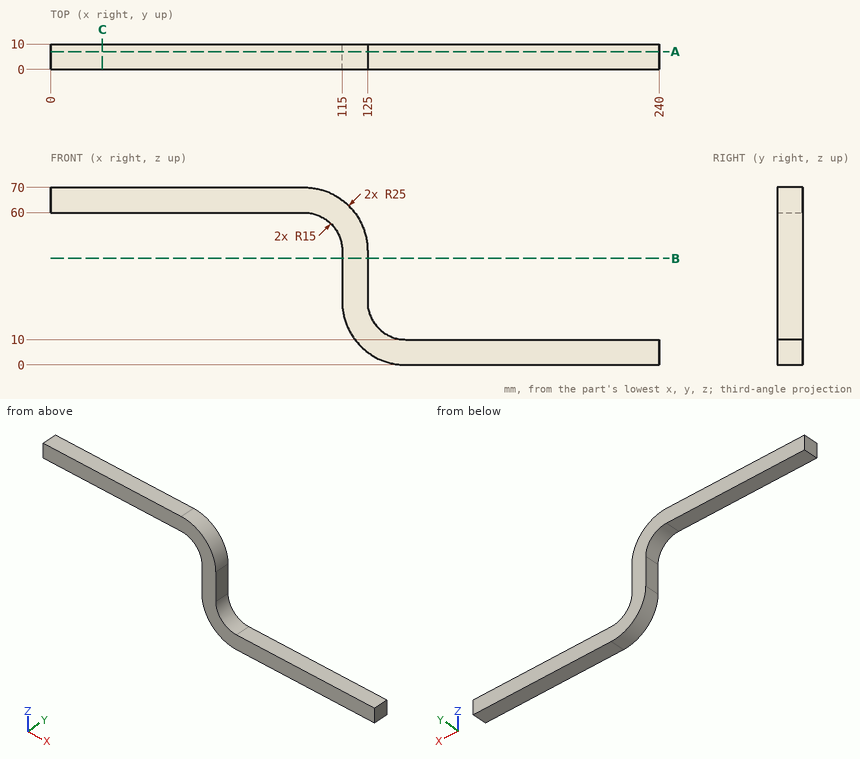
Source: three-view drawing plus pictorial views. Frame: mm from the lowest corner of the part. Round coordinates to 2 decimals unless told otherwise and drop trailing zeros. Loops run counter-clockwise (first coordinate to the right, second up) from the corner with the lowest first, then second, coordinate; pieces in that order, holes last. Notation, with made-up numbers: (75.25, 50) -> (108.25, 50) arc R29 ccw to (108.25, 89) -> close; hole circle Ø2 at (-27, 78). An arc over 180 degrees is marked (long way). Use one line per item in the form item = value.
Item 1: Material intervals for probe 1 along Z at (x, y) = (192, 4.25); probe 2 along Z at (x, y) = (81, 1.5); probe 3 along X at (y, z) = (3, 28), sorted ascending.
Evaluation:
probe_1 = 0 to 10
probe_2 = 60 to 70
probe_3 = 115 to 125
Item 2: Contact query for flat-ended pins moving along their axis: pin 1 Ø2 at (x, y) = (92.5, 5) entering from -Z; pin 2 Ø3 at (y, z) = (5.5, 34.5) entering from +X; pin 3 Ø2 at (x, y) = (149, 2.5) entering from +Z. Output: stop coordinate, or through.
Evaluation:
pin_1 = 60
pin_2 = 125
pin_3 = 10
Item 3: Cut plane B-B on z = 42. Output: boundary loops of the cut face in (x, y).
Evaluation:
outline = (115, 0) -> (125, 0) -> (125, 10) -> (115, 10) -> close
Item 4: Cut plane A-A on y = 7. Output: boundary loops of the cut face in (x, z).
Evaluation:
outline = (0, 60) -> (100, 60) arc R15 cw to (115, 45) -> (115, 25) arc R25 ccw to (140, 0) -> (240, 0) -> (240, 10) -> (140, 10) arc R15 cw to (125, 25) -> (125, 45) arc R25 ccw to (100, 70) -> (0, 70) -> close
Item 5: Cut plane C-C on x = 20.5. Output: boundary loops of the cut face in (y, z), then the cut area to 3 significant figures.
Evaluation:
outline = (0, 60) -> (10, 60) -> (10, 70) -> (0, 70) -> close
area = 100 mm2
